Could you check a few things on this model? Use its own coordinates, in mm. Round coordinates to 2 decimals unless told otherwise and drop trailing zeros. Loops run counter-clockwise (first coordinate to the right, second up) from the corner with the lowest first, then second, coordinate; pieces in that order, holes last. Notation, with made-up numbers: (-25, 71) -> (-7, 71) arc R8 cw to (-7, 80) -> close; hole circle Ø11 at (18.5, 70). An arc over 180 degrees is marked (long way). Put each result on its own line as item: value. Start each with the question number.
1. If we mould it in two halves opening along Z, with no side actions, what happens to faces 1 (the flat face through (0, 0, 0)), 2 (the cylindrical face through (0.084, -5.699, 4.715)), 3 (the flat face through (0, 6, 2))? For each: pulls with the +Z half, pulls with the -Z half, needs draft (parallel to the pull), parting line crosses it, or undercut.
2. I'm going to push a flat-ended pin straight in: P1, Ø3, axis at y = 2.5, z = 1.5, coming from the +X side. Where does the tip first touch, or does it pass through?
3. I need wall thicknesses on line 1 (X direction, y = -0.25, z = 1.5); line 2 (X direction, y = 3.75, z = 3.7); line 3 (Y direction, x = -6.75, z = 4.5). Which ranges of each line are inside material? Lowest first, please. Write a range as [from, to].
4. Imagine slicing it at A-A, the plane z = 0.3. Please give me the cut outline in (x, y).
Autodesk Inventor part; units mm, degrees
ref_plane "YZ Plane" through (0, 0, 0) normal (1, 0, 0) x (0, 1, 0)
ref_plane "XZ Plane" through (0, 0, 0) normal (0, 1, 0) x (-1, 0, 0)
ref_plane "XY Plane" through (0, 0, 0) normal (0, 0, 1) x (1, 0, 0)
sketch "Sketch1" plane through (0, 0, 0) normal (0, 0, 1) x (1, 0, 0)
  line L0 (-14.4, 0) -> (2.4, 0)
  line L1 (0, -8.4) -> (0, 8.4)
  line L2 (0, 6) -> (-6, 6)
  line L3 (-6, 6) -> (-6, -6)
  line L4 (-6, -6) -> (0, -6)
  line L5 (0, -6) -> (0, 6)
  arc A0 (-6, 6) -> (-6, -6) centre (-6, 0) ccw
  point P0 (0, 0)
  dimension "d0" = 12
  dimension "d1" = 6
extrude "Extrusion1" add sketch "Sketch1" along normal blind 5
fillet "Fillet1" radius 1 3 edges at (-3, -6, 5) (-3, 6, 5) (-12, 0, 5)
mirror "Mirror1" about plane through (0, -6, 0) normal (1, 0, 0)
properties part number "F113" material "ABS Plastic"
Entries:
1. face 1: pulls with the -Z half
1. face 2: pulls with the +Z half
1. face 3: needs draft
2. P1: x = 11.92
3. line 1: [-11.99, 11.99]
3. line 2: [-10.68, 10.68]
3. line 3: [-5.82, 5.82]
4. outline: (-6, -6) -> (6, -6) arc R6 ccw to (6, 6) -> (-6, 6) arc R6 ccw to start
